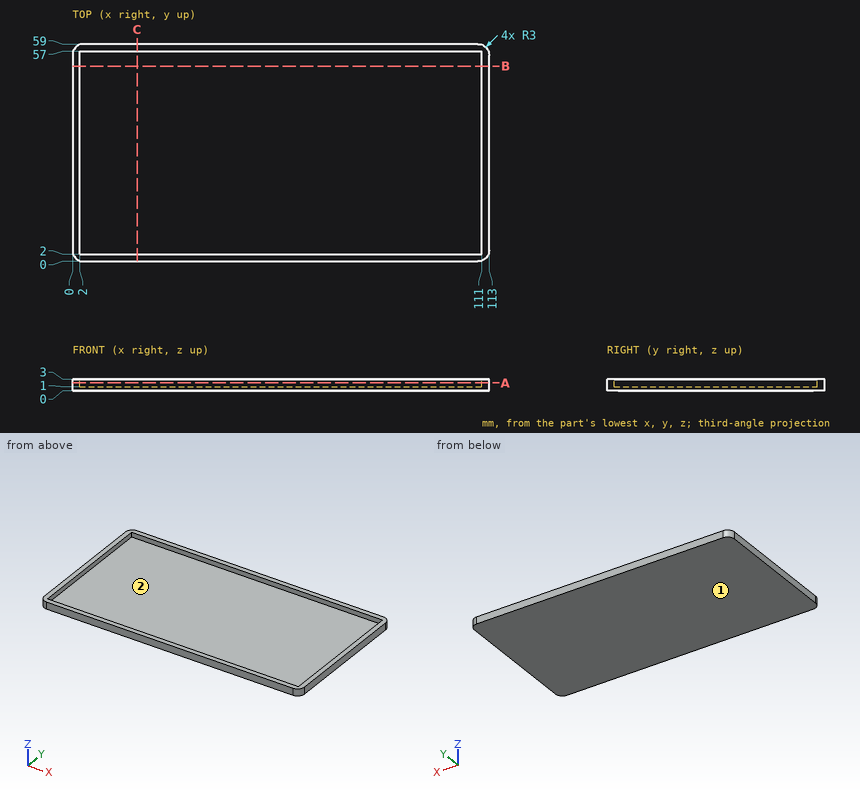
The figure shows three views and two pictorial views of one solid part (mm, origin at its lowest corner). Answer the questions. Give positions to 0.01 mm unless a question says otherwise; leave off trailing zeros. Order: outer loops, then holes, each group sorted by start corner. A loop starts at its lowest first (then second) coordinate and runs counter-clockwise, first axis right, second up. Notation, with made-up numbers: (-20.5, 29) -> (37.5, 29) arc R29 ccw to (37.5, 65) -> close; hole circle Ø8 at (18.25, 75). An arc over 180 degrees is marked (long way). One line per item, written item: value.
1) Determine the mould class of the marked faces 1 and 2 for opening direction Y: pulls with the +Y half, pulls with the -Y half, needs draft (parallel to the pull), parting line crosses it, or undercut.
Reported:
face 1: needs draft
face 2: undercut
2) A flat-ended cylindrical pin translates along its axis: P1, Ø6, axis at x = 60.5, y = 38.5, coming from the -Z side. Find the tip coordinate at first contact, or state that the pin passes through.
Reported:
P1: stops at z = 0
3) Find section B-B, the plane y = 53. Determine the outline of the cut face in (x, z), plus the area to 3 significant figures.
Reported:
outline: (0, 0) -> (113, 0) -> (113, 3) -> (111, 3) -> (111, 1) -> (2, 1) -> (2, 3) -> (0, 3) -> close
area: 121 mm^2
4) Find the intervals of material crossed by line 1 (Y direction, x = 11, z = 1.1); line 2 (X direction, y = 15, z = 1.65); line 3 (Z direction, x = 6, y = 51.5), in increasing order.
Reported:
line 1: y = 0 to 2, 57 to 59
line 2: x = 0 to 2, 111 to 113
line 3: z = 0 to 1
5) Find section C-C, the plane x = 17.5. Determine the outline of the cut face in (y, z).
Reported:
outline: (0, 0) -> (59, 0) -> (59, 3) -> (57, 3) -> (57, 1) -> (2, 1) -> (2, 3) -> (0, 3) -> close
6) Find section A-A, the plane z = 2.05. Determine the outline of the cut face in (x, y).
Reported:
outline: (0, 3) arc R3 ccw to (3, 0) -> (110, 0) arc R3 ccw to (113, 3) -> (113, 56) arc R3 ccw to (110, 59) -> (3, 59) arc R3 ccw to (0, 56) -> close; hole (2, 2) -> (111, 2) -> (111, 57) -> (2, 57) -> close
